Build history of the part. All positions in model axes, mm. A direction names the side the tool comes from. Round coordinates to 2 decimals unless told otherwise and drop trailing zeros. Write each loop counter-clockwise with the first axis right and the second up, starting at its lowest first coordinate (ties: lowest second). Pieces come first, ordered by that corner, then holes. Notation, with made-up numbers: (39.5, 32.5) - (97.5, 32.5) arc R12 ccw to (97.5, 49.5) - close; hole circle Ø7 at (-36, 82). An arc over 180 degrees is marked (long way). Answer as a JSON object with one key per item and string values. Group by question number.
Item 1: Slice it at B-B, the plane z = 121.5. List the corners of the cut face in (x, y).
Item 2: Slice it at C-C, the plane y = 2.75. List the corners of the cut face in (x, z).
Item 3: Slice it at A-A, the plane x = 6.5. List the corners of the cut face in (y, z).
Item 4: Which spindle directions (+Z, -Z, +X, -X, +Y, -Y) get a long thin tool onto all of the face, cutting with end or side? Do faces 1 (the flat face through (23.818, -1, 113)), 2 (the flat face through (-1, -11, 228.6)). Say none if no direction does.
Item 5: Probe line 1 (X direction, y = 11.65, z = 165.1); line 2 (X direction, y = -9.75, z = 160); line 3 (Y direction, x = 6, z = 67.5). List the from-to ranges inside material, lowest first. Write a range as from..to.
Item 6: Two-plate mould, pull along Y, no slides. Class faces 3 (the flat face through (26.358, -1, 113)), 4 (the flat face through (1, 12.28, 113)), 5 (the flat face through (1, 9.74, 113)), 6 (the flat face through (1, -13.12, 113)): +Y half, -Y half, draft (parallel to the pull), parting line (faces both ways), or undercut.
from build123d import *

# Parameters (mm, degrees)
SKETCH1_W               = 50.8
SKETCH1_H               = 25.4
SKETCH1_W_2             = 45.72
SKETCH1_H_2             = 20.32
BOSS_EXTRUDE1_DEPTH     = 228.6
SKETCH2_R               = 0.5
CUT_EXTRUDE1_DEPTH      = 1
CUT_EXTRUDE1_DEPTH_BACK = 26.4


with BuildPart() as part:
    # Sketch1 → Boss-Extrude1 (new body)
    with BuildSketch(Plane.XY):
        with Locations((0.958397508, -0.419684268)):
            Rectangle(SKETCH1_W, SKETCH1_H)
        with Locations((0.958397508, -0.419684268)):
            Rectangle(SKETCH1_W_2, SKETCH1_H_2, mode=Mode.SUBTRACT)
    extrude(amount=BOSS_EXTRUDE1_DEPTH)

    # Sketch2 → Cut-Extrude1 (cut, two sides)
    with BuildSketch(Plane(origin=(0, 12.280315732, 0), x_dir=(1, 0, 0), z_dir=(0, 1, 0))) as cut_extrude1_sk:
        with Locations((-11.741602492, -215.9)):
            Circle(SKETCH2_R)
        with Locations((0.958397508, -215.9)):
            Circle(SKETCH2_R)
        with Locations((13.658397508, -215.9)):
            Circle(SKETCH2_R)
        with Locations((0.958397508, -203.2)):
            Circle(SKETCH2_R)
        with Locations((13.658397508, -203.2)):
            Circle(SKETCH2_R)
        with Locations((0.958397508, -190.5)):
            Circle(SKETCH2_R)
        with Locations((13.658397508, -190.5)):
            Circle(SKETCH2_R)
        with Locations((0.958397508, -177.8)):
            Circle(SKETCH2_R)
        with Locations((13.658397508, -177.8)):
            Circle(SKETCH2_R)
        with Locations((0.958397508, -165.1)):
            Circle(SKETCH2_R)
        with Locations((13.658397508, -165.1)):
            Circle(SKETCH2_R)
        with Locations((0.958397508, -152.4)):
            Circle(SKETCH2_R)
        with Locations((13.658397508, -152.4)):
            Circle(SKETCH2_R)
        with Locations((0.958397508, -139.7)):
            Circle(SKETCH2_R)
        with Locations((13.658397508, -139.7)):
            Circle(SKETCH2_R)
        with Locations((0.958397508, -127)):
            Circle(SKETCH2_R)
        with Locations((13.658397508, -127)):
            Circle(SKETCH2_R)
        with Locations((0.958397508, -114.3)):
            Circle(SKETCH2_R)
        with Locations((13.658397508, -114.3)):
            Circle(SKETCH2_R)
        with Locations((0.958397508, -101.6)):
            Circle(SKETCH2_R)
        with Locations((13.658397508, -101.6)):
            Circle(SKETCH2_R)
        with Locations((0.958397508, -88.9)):
            Circle(SKETCH2_R)
        with Locations((13.658397508, -88.9)):
            Circle(SKETCH2_R)
        with Locations((0.958397508, -76.2)):
            Circle(SKETCH2_R)
        with Locations((13.658397508, -76.2)):
            Circle(SKETCH2_R)
        with Locations((0.958397508, -63.5)):
            Circle(SKETCH2_R)
        with Locations((13.658397508, -63.5)):
            Circle(SKETCH2_R)
        with Locations((0.958397508, -50.8)):
            Circle(SKETCH2_R)
        with Locations((13.658397508, -50.8)):
            Circle(SKETCH2_R)
        with Locations((0.958397508, -38.1)):
            Circle(SKETCH2_R)
        with Locations((13.658397508, -38.1)):
            Circle(SKETCH2_R)
        with Locations((0.958397508, -25.4)):
            Circle(SKETCH2_R)
        with Locations((13.658397508, -25.4)):
            Circle(SKETCH2_R)
        with Locations((0.958397508, -12.7)):
            Circle(SKETCH2_R)
        with Locations((13.658397508, -12.7)):
            Circle(SKETCH2_R)
        with Locations((-11.741602492, -203.2)):
            Circle(SKETCH2_R)
        with Locations((-11.741602492, -190.5)):
            Circle(SKETCH2_R)
        with Locations((-11.741602492, -177.8)):
            Circle(SKETCH2_R)
        with Locations((-11.741602492, -165.1)):
            Circle(SKETCH2_R)
        with Locations((-11.741602492, -152.4)):
            Circle(SKETCH2_R)
        with Locations((-11.741602492, -139.7)):
            Circle(SKETCH2_R)
        with Locations((-11.741602492, -127)):
            Circle(SKETCH2_R)
        with Locations((-11.741602492, -114.3)):
            Circle(SKETCH2_R)
        with Locations((-11.741602492, -101.6)):
            Circle(SKETCH2_R)
        with Locations((-11.741602492, -88.9)):
            Circle(SKETCH2_R)
        with Locations((-11.741602492, -76.2)):
            Circle(SKETCH2_R)
        with Locations((-11.741602492, -63.5)):
            Circle(SKETCH2_R)
        with Locations((-11.741602492, -50.8)):
            Circle(SKETCH2_R)
        with Locations((-11.741602492, -38.1)):
            Circle(SKETCH2_R)
        with Locations((-11.741602492, -25.4)):
            Circle(SKETCH2_R)
        with Locations((-11.741602492, -12.7)):
            Circle(SKETCH2_R)
    extrude(amount=CUT_EXTRUDE1_DEPTH, mode=Mode.SUBTRACT)
    extrude(cut_extrude1_sk.sketch, amount=-CUT_EXTRUDE1_DEPTH_BACK, mode=Mode.SUBTRACT)


solid = part.part
Geometry says:
{
 "1": {"outline": "(-24.44, -13.12) - (26.36, -13.12) - (26.36, 12.28) - (-24.44, 12.28) - close; hole (-21.9, -10.58) - (23.82, -10.58) - (23.82, 9.74) - (-21.9, 9.74) - close"},
 "2": {"outline": "(-24.44, 0) - (-21.9, 0) - (-21.9, 228.6) - (-24.44, 228.6) - close; (23.82, 0) - (26.36, 0) - (26.36, 228.6) - (23.82, 228.6) - close"},
 "3": {"outline": "(-13.12, 0) - (-10.58, 0) - (-10.58, 228.6) - (-13.12, 228.6) - close; (9.74, 0) - (12.28, 0) - (12.28, 228.6) - (9.74, 228.6) - close"},
 "4": {"face 1": "+Z, -Z", "face 2": "+Z, +X, -X, +Y, -Y"},
 "5": {"line 1": "x = -24.44..-12.24, -11.24..0.46, 1.46..13.16, 14.16..26.36", "line 2": "x = -24.44..-21.9, 23.82..26.36", "line 3": "y = -13.12..-10.58, 9.74..12.28"},
 "6": {"face 3": "draft", "face 4": "+Y half", "face 5": "undercut", "face 6": "-Y half"}
}
